Here's how the part is built. I have some questions about the finished solid (model axes, mm). Face numbers are marked on the shaded views. A direction names the side the tool comes from. Round coordinates to 2 decimals unless told otherwise and drop trailing zeros. Order: outer loops, then holes, each group sorted by start corner. A loop starts at its lowest first (then second) coordinate and runs counter-clockwise, first axis right, second up. Notation, with made-up numbers: (26.5, -9.75) -> (84.5, -9.75) arc R30 ccw to (84.5, 23.25) -> close; hole circle Ø1 at (-28.5, 81). An arc over 180 degrees is marked (long way). Use a Markdown table: item, result. Add a question column.
(1) If I drill on probe 1 along Y at (x, z) = (16.25, -23); probe 2 along Z at (x, y) = (8.89, -54.25); probe 3 along Y at (x, z) = (-3.3, 13.97), over which ranges is the centre line in solid material (lowest first)?
(2) I want a section at B-B, the plane z = 10.16. Please give me the cut outline in (x, y), then the cut area to 3 significant figures.
(3) On a 3-axis mill with a long thin cutter (end or side, diameter ignored), from which of +Z, -Z, +X, -X, +Y, -Y can I reach the whole of each face in a straight line? I mean the marked faces 4, 5, 6 and 7. Say none if no direction works.
(4) Thinking about a two-plate mould opening in Y: for the marked faces 1, 2 and 3, which applies, pulls with the +Y half, pulls with the -Y half, needs draft (parallel to the pull), parting line crosses it, or undercut?
(5) I'm going to push flat-ended pins straight in: P1, Ø4.5, axis at x = 8.89, z = -15.24, coming from the +Y side; P2, Ø4, axis at x = 8.89, z = 15.24, coming from the -Y side; P3, Ø1.5, axis at x = 12.7, z = -10.16, coming from the +Y side; P4, Ø10.5, axis at y = -2.5, z = -4.5, coming from the +X side. Where does each tip first touch, or does it pass through?
(6) I want a section at C-C, the plane y = 10. Please give me the cut outline in (x, z).
(7) I want a section at D-D, the plane z = 0. Please give me the cut outline in (x, y), then the cut area to 3 significant figures.
(8) I want a section at A-A, the plane x = 8.89. Please give me the cut outline in (y, z).
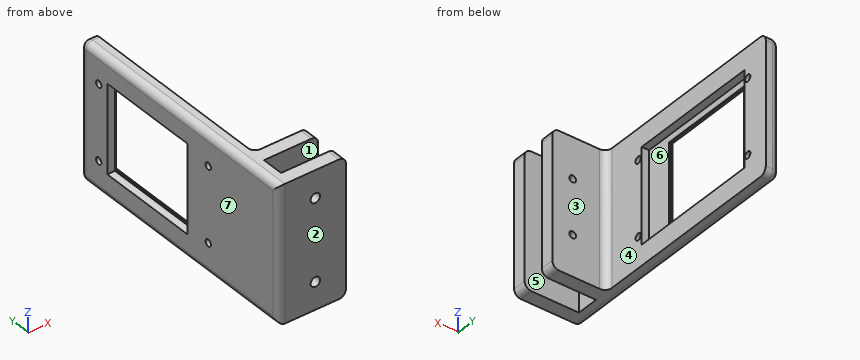
from build123d import *
from OCP.BRepFilletAPI import BRepFilletAPI_MakeChamfer

# Parameters (mm, degrees)
BOSS_EXTRUDE7_DEPTH = 25.4
SKETCH14_W          = 30.48
SKETCH14_H          = 36.068
CUT_EXTRUDE3_DEPTH  = 66.482787481
SKETCH15_W          = 35.56
SKETCH15_H          = 49.53
CUT_EXTRUDE4_DEPTH  = 2.794
CHAMFER1_SIZE       = 1.778
CHAMFER1_SIZE2      = 1.244969003
SKETCH16_R          = 1.27
CUT_EXTRUDE5_DEPTH  = 66.482787481
FILLET4_R           = 2.54
FILLET5_R           = 2.54
SKETCH23_R          = 1.778
CUT_EXTRUDE6_DEPTH  = 96.857661666
FILLET6_R           = 2.54
CUT_EXTRUDE7_REACH  = 85.437
SKETCH24_R          = 1.27
FILLET7_R           = 2.54


with BuildPart() as part:
    # Sketch12 → Boss-Extrude7 (new, symmetric)
    with BuildSketch(Plane.XY):
        Polygon((0, -38.4175), (20.32, -38.4175), (20.32, -43.4975), (0, -43.4975), (0, -51.7525), (20.32, -51.7525), (20.32, -56.8325), (-5.08, -56.8325), (-5.08, 38.4175), (0, 38.4175), align=None)
    extrude(amount=BOSS_EXTRUDE7_DEPTH, both=True)

    # Sketch14 → Cut-Extrude3 (cut, through all)
    with BuildSketch(Plane(origin=(0, 0, 0), x_dir=(0, 0, -1), z_dir=(1, 0, 0))):
        with Locations((0, 6.2103)):
            Rectangle(SKETCH14_W, SKETCH14_H)
    extrude(amount=-CUT_EXTRUDE3_DEPTH, mode=Mode.SUBTRACT)

    # Sketch15 → Cut-Extrude4 (cut)
    with BuildSketch(Plane(origin=(0, 0, 0), x_dir=(0, 0, -1), z_dir=(1, 0, 0))):
        with Locations((0, 3.2893)):
            Rectangle(SKETCH15_W, SKETCH15_H)
    extrude(amount=-CUT_EXTRUDE4_DEPTH, mode=Mode.SUBTRACT)

    # Chamfer1: one chamfer whose edges measure the first distance from different faces: ONE call of the kernel's chamfer builder (chamfer() names one face for all edges)
    chamfer1_edges_1 = [part.edges().sort_by_distance(p)[0] for p in [
        (-5.08, 6.2103, -15.24),
    ]]
    chamfer1_side_1 = [part.faces().sort_by_distance(p)[0] for p in [
        (-3.937, 6.2103, -15.24),
    ]]
    chamfer1_edges_2 = [part.edges().sort_by_distance(p)[0] for p in [
        (-5.08, -11.8237, 0),
    ]]
    chamfer1_side_2 = [part.faces().sort_by_distance(p)[0] for p in [
        (-3.937, -11.8237, 0),
    ]]
    chamfer1_edges_3 = [part.edges().sort_by_distance(p)[0] for p in [
        (-5.08, 6.2103, 15.24),
    ]]
    chamfer1_side_3 = [part.faces().sort_by_distance(p)[0] for p in [
        (-3.937, 6.2103, 15.24),
    ]]
    chamfer1_edges_4 = [part.edges().sort_by_distance(p)[0] for p in [
        (-5.08, 24.2443, 0),
    ]]
    chamfer1_side_4 = [part.faces().sort_by_distance(p)[0] for p in [
        (-3.937, 24.2443, 0),
    ]]
    chamfer1 = BRepFilletAPI_MakeChamfer(part.part.solid().wrapped)
    for e in chamfer1_edges_1:
        chamfer1.Add(CHAMFER1_SIZE, CHAMFER1_SIZE2, e.wrapped, chamfer1_side_1[0].wrapped)  # the first distance lies on this face
    for e in chamfer1_edges_2:
        chamfer1.Add(CHAMFER1_SIZE, CHAMFER1_SIZE2, e.wrapped, chamfer1_side_2[0].wrapped)  # the first distance lies on this face
    for e in chamfer1_edges_3:
        chamfer1.Add(CHAMFER1_SIZE, CHAMFER1_SIZE2, e.wrapped, chamfer1_side_3[0].wrapped)  # the first distance lies on this face
    for e in chamfer1_edges_4:
        chamfer1.Add(CHAMFER1_SIZE, CHAMFER1_SIZE2, e.wrapped, chamfer1_side_4[0].wrapped)  # the first distance lies on this face
    add(Compound.cast(chamfer1.Shape()), mode=Mode.REPLACE)

    # Sketch16 → Cut-Extrude5 (cut, through all)
    with BuildSketch(Plane(origin=(0, 0, 0), x_dir=(0, 0, -1), z_dir=(1, 0, 0))):
        with Locations((-13.97, 29.7053)):
            Circle(SKETCH16_R)
        with Locations((13.97, 29.7053)):
            Circle(SKETCH16_R)
        with Locations((-13.97, -23.1267)):
            Circle(SKETCH16_R)
        with Locations((13.97, -23.1267)):
            Circle(SKETCH16_R)
    extrude(amount=-CUT_EXTRUDE5_DEPTH, mode=Mode.SUBTRACT)

    # Fillet4
    fillet4_edges = [part.edges().sort_by_distance(p)[0] for p in [
        (-2.54, 38.4175, 25.4),
        (-2.54, 38.4175, -25.4),
    ]]
    fillet(fillet4_edges, radius=FILLET4_R)

    # Fillet5
    fillet5_edges = [part.edges().sort_by_distance(p)[0] for p in [
        (20.32, -54.2925, 25.4),
        (20.32, -40.9575, -25.4),
        (20.32, -54.2925, -25.4),
        (20.32, -40.9575, 25.4),
    ]]
    fillet(fillet5_edges, radius=FILLET5_R)

    # Sketch23 → Cut-Extrude6 (cut, through all)
    with BuildSketch(Plane(origin=(0, -51.7525, 0), x_dir=(1, 0, 0), z_dir=(0, 1, 0))):
        with Locations(Location((8.89, 15.24, 0), (0, 0, 180))):
            Circle(SKETCH23_R)
        with Locations(Location((8.89, -15.24, 0), (0, 0, 180))):
            Circle(SKETCH23_R)
    extrude(amount=-CUT_EXTRUDE6_DEPTH, mode=Mode.SUBTRACT)

    # Fillet6
    fillet6_edges = [part.edges().sort_by_distance(p)[0] for p in [
        (-5.08, -56.8325, 0),
        (-5.08, 38.4175, 0),
        (-5.08, -10.4775, -25.4),
        (-5.08, -10.4775, 25.4),
        (-5.08, 37.673551224, 24.656051224),
        (-5.08, 37.673551224, -24.656051224),
    ]]
    fillet(fillet6_edges, radius=FILLET6_R)

    # Sketch24 → Cut-Extrude7 (cut, up to next)
    with BuildSketch(Plane(origin=(0, -38.4175, 0), x_dir=(1, 0, 0), z_dir=(0, 1, 0)), mode=Mode.PRIVATE) as cut_extrude7_sk1:
        with Locations(Location((12.7, 10.16, 0), (0, 0, 180))):
            Circle(SKETCH24_R)
    cut_extrude7_tool1 = extrude(cut_extrude7_sk1.sketch, amount=-CUT_EXTRUDE7_REACH, mode=Mode.PRIVATE) & part.part
    # Sketch24 → Cut-Extrude7 (cut, up to next)
    with BuildSketch(Plane(origin=(0, -38.4175, 0), x_dir=(1, 0, 0), z_dir=(0, 1, 0)), mode=Mode.PRIVATE) as cut_extrude7_sk2:
        with Locations(Location((12.7, -10.16, 0), (0, 0, 180))):
            Circle(SKETCH24_R)
    cut_extrude7_tool2 = extrude(cut_extrude7_sk2.sketch, amount=-CUT_EXTRUDE7_REACH, mode=Mode.PRIVATE) & part.part
    add(cut_extrude7_tool1.solids().sort_by_distance((12.7, -38.4175, -10.16))[0], mode=Mode.SUBTRACT)
    add(cut_extrude7_tool2.solids().sort_by_distance((12.7, -38.4175, 10.16))[0], mode=Mode.SUBTRACT)

    # Fillet7
    fillet7_edges = [part.edges().sort_by_distance(p)[0] for p in [
        (0, -38.4175, 0),
    ]]
    fillet(fillet7_edges, radius=FILLET7_R)


solid = part.part
Taken from the geometry:
| question | item | result |
|---|---|---|
| 1 | probe 1 | y = -56.83 to -51.75, -43.5 to -38.42 |
| 1 | probe 2 | z = -25.4 to -17.02, -13.46 to 13.46, 17.02 to 25.4 |
| 1 | probe 3 | y = -56.72 to -24.4, -21.86 to -11.82, 24.24 to 28.44, 30.98 to 38.3 |
| 2 | outline | (-5.08, -54.29) arc R2.54 ccw to (-2.54, -56.83) -> (20.32, -56.83) -> (20.32, -51.75) -> (0, -51.75) -> (0, -43.5) -> (11.43, -43.5) -> (11.43, -38.42) -> (2.54, -38.42) arc R2.54 cw to (0, -35.88) -> (0, -21.48) -> (-2.79, -21.48) -> (-2.79, -11.82) -> (-3.3, -11.82) -> (-5.08, -13.07) -> close; (-5.08, 25.49) -> (-3.3, 24.24) -> (-2.79, 24.24) -> (-2.79, 28.05) -> (0, 28.05) -> (0, 38.42) -> (-2.54, 38.42) arc R2.54 ccw to (-5.08, 35.88) -> close; (13.97, -43.5) -> (20.32, -43.5) -> (20.32, -38.42) -> (13.97, -38.42) -> close |
| 2 | area | 453 mm2 |
| 3 | face 4 | +Z, -Z, +X, +Y |
| 3 | face 5 | +Z, -Z, +X |
| 3 | face 6 | +X |
| 3 | face 7 | +Z, -Z, -X, +Y, -Y |
| 4 | face 1 | undercut |
| 4 | face 2 | pulls with the -Y half |
| 4 | face 3 | pulls with the +Y half |
| 5 | P1 | stops at y = -38.42 |
| 5 | P2 | stops at y = -56.83 |
| 5 | P3 | stops at y = -51.75 |
| 5 | P4 | passes through |
| 6 | outline | (-5.08, -22.86) arc R2.54 ccw to (-2.54, -25.4) -> (0, -25.4) -> (0, -17.78) -> (-2.79, -17.78) -> (-2.79, -15.24) -> (-3.3, -15.24) -> (-5.08, -16.48) -> close; (-5.08, 16.48) -> (-3.3, 15.24) -> (-2.79, 15.24) -> (-2.79, 17.78) -> (0, 17.78) -> (0, 25.4) -> (-2.54, 25.4) arc R2.54 ccw to (-5.08, 22.86) -> close |
| 7 | outline | (-5.08, -54.29) arc R2.54 ccw to (-2.54, -56.83) -> (20.32, -56.83) -> (20.32, -51.75) -> (0, -51.75) -> (0, -43.5) -> (20.32, -43.5) -> (20.32, -38.42) -> (2.54, -38.42) arc R2.54 cw to (0, -35.88) -> (0, -21.48) -> (-2.79, -21.48) -> (-2.79, -11.82) -> (-3.3, -11.82) -> (-5.08, -13.07) -> close; (-5.08, 25.49) -> (-3.3, 24.24) -> (-2.79, 24.24) -> (-2.79, 28.05) -> (0, 28.05) -> (0, 38.42) -> (-2.54, 38.42) arc R2.54 ccw to (-5.08, 35.88) -> close |
| 7 | area | 466 mm2 |
| 8 | outline | (-56.83, -25.4) -> (-51.75, -25.4) -> (-51.75, -17.02) -> (-56.83, -17.02) -> close; (-56.83, -13.46) -> (-51.75, -13.46) -> (-51.75, 13.46) -> (-56.83, 13.46) -> close; (-56.83, 17.02) -> (-51.75, 17.02) -> (-51.75, 25.4) -> (-56.83, 25.4) -> close; (-43.5, -25.4) -> (-38.42, -25.4) -> (-38.42, 25.4) -> (-43.5, 25.4) -> close |
